Here's how the part is built. I have some questions about the finished solid (model axes, mm). Face numbers are marked on the shaded views. Coordinates: 2 decimals unless noted, no trailing zeros. Use one line per item in the form item = value. Start each with the question number.
1. Please list where these lines run through material, in increasing order: line 1 along Y through (x, z) = (0, 28); line 2 along Y through (x, z) = (-21, 58.5); line 3 along Z through (x, y) = (0, -47). Write a range as [from, to].
2. I'm going to push flat-ended pins straight in: pin 1 Ø3 at (x, z) = (-18.5, 33.5) entering from +Y; pin 2 Ø10 at (x, z) = (44.5, 45) entering from +Y; pin 3 Ø2 at (x, z) = (-17.5, 86.5) entering from +Y; pin 4 Ø4 at (x, z) = (47.5, 24) entering from -Y. Where does each tip first touch, or does it pass through?
3. Thinking about a two-plate mould opening in Y: for the marked faces 1, 2 and 3, which applies, released by +Y, released by -Y, zero draft, split by the parting line, or undercut?
from build123d import *


with BuildPart() as f1:
    # F0 (on Front) → F1 (revolve)
    with BuildSketch(Plane.XZ):
        with BuildLine():
            Line((7.9375, 101.6), (7.9375, 0))
            Line((7.9375, 0), (41.275, 0))
            ThreePointArc((41.275, 0), (43.520064, 0.929936), (44.45, 3.175))
            Line((44.45, 3.175), (44.45, 73.976143))
            ThreePointArc((44.45, 73.976143), (45.024461, 75.797632), (46.539966, 76.959988))
            Line((46.539966, 76.959988), (61.9125, 82.55))
            Line((61.9125, 82.55), (61.9125, 98.425))
            Line((61.9125, 98.425), (61.9125, 101.6))
            Line((61.9125, 101.6), (58.7375, 101.6))
            Line((58.7375, 101.6), (7.9375, 101.6))
        make_face()
    revolve(axis=Axis((0, 0, 44.177184), (0, 0, 1)))


solid = f1.part
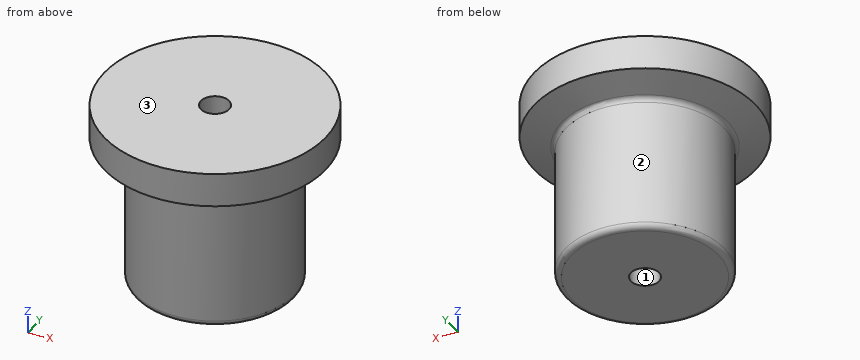
Answer list:
q1.line_1 = [-44.45, -7.94], [7.94, 44.45]
q1.line_2 = [-39.18, 39.18]
q1.line_3 = [77.13, 101.6]
q2.pin_1 = 41.07
q2.pin_2 = 20.39
q2.pin_3 = 59.67
q2.pin_4 = through
q3.face_1 = undercut
q3.face_2 = split by the parting line
q3.face_3 = zero draft
